The figure shows three views and two pictorial views of one solid part (mm, origin at its lowest corner). Answer the questions. Coordinates: 2 decimals unless noted, no trailing zeros. Order: outer loops, then holes, each group sorted by start corner. A loop starts at its lowest first (then second) coordinate and runs counter-clockwise, first axis right, second up. Notation, with made-up numbers: M 75,57.5 L 119,57.5 A10 ccw 119,68.5 Z; hole C -9.75,-30.75 d1. An arc over 180 degrees is marked long. Use a Markdown table: item, result.
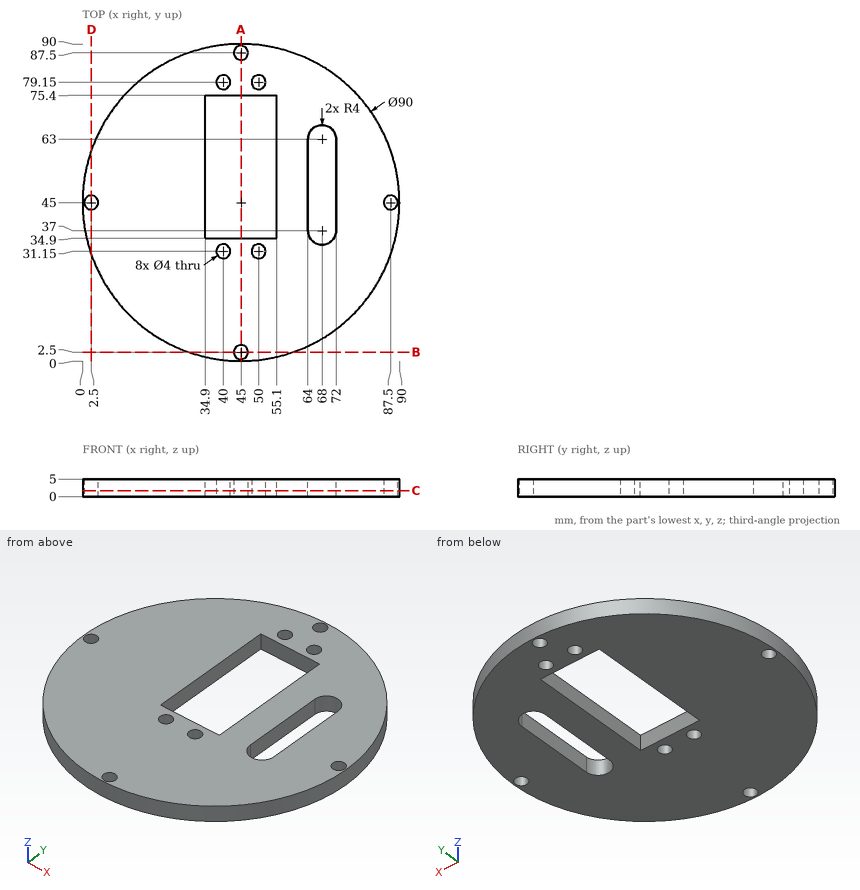
1. Find the intervals of material crossed by probe 1 along Y at (x, z) = (45, 1.55); probe 2 along Y at (x, z) = (49.5, 2.9); probe 3 along X at (y, z) = (35, 1.6), in increasing order.
Answers below:
| item | result |
|---|---|
| probe 1 | 0 to 0.5, 4.5 to 34.9, 75.4 to 85.5, 89.5 to 90 |
| probe 2 | 0.23 to 29.21, 33.09 to 34.9, 75.4 to 77.21, 81.09 to 89.77 |
| probe 3 | 1.13 to 34.9, 55.1 to 64.54, 71.46 to 88.87 |
2. Section A-A on x = 45 is taken. Determine the outline of the cut face in (y, z).
Answers below:
| item | result |
|---|---|
| outline | M 0,0 L 0.5,0 L 0.5,5 L 0,5 Z; M 4.5,0 L 34.9,0 L 34.9,5 L 4.5,5 Z; M 75.4,0 L 85.5,0 L 85.5,5 L 75.4,5 Z; M 89.5,0 L 90,0 L 90,5 L 89.5,5 Z |
3. Flat-ended cylindrical pins translate along their axes: P1, Ø1.5, axis at y = 48.5, z = 4.5, coming from the +X side; P2, Ø3.5, axis at x = 2.5, y = 45, coming from the -Z side; P3, Ø10, axis at x = 50, y = 13.5, coming from the -Z side; P4, Ø1.5, axis at y = 71, z = 1, coming from the +X side. Find the tip coordinate at first contact, or state that the pin passes through.
Answers below:
| item | result |
|---|---|
| P1 | x = 89.92 |
| P2 | through |
| P3 | z = 0 |
| P4 | x = 82.25 |
4. Section B-B on y = 2.5 is taken. Determine the outline of the cut face in (x, z).
Answers below:
| item | result |
|---|---|
| outline | M 30.21,0 L 43,0 L 43,5 L 30.21,5 Z; M 47,0 L 59.79,0 L 59.79,5 L 47,5 Z |
5. Section C-C on z = 1.7 is taken. Give the number of separate pieces and of enclosed holes in the cut face, then the cut area to 3 significant figures.
Answers below:
| item | result |
|---|---|
| separate pieces | 1 |
| enclosed holes | 10 |
| area | 5,180 mm² |
